from build123d import *

# Parameters (mm, degrees)
SKETCH1_R           = 3.4036
BOSS_EXTRUDE1_DEPTH = 304.8


with BuildPart() as part:
    # Sketch1 → Boss-Extrude1 (new body, symmetric)
    with BuildSketch(Plane.XY):
        with BuildLine():
            Line((-39.878, 16.891), (-39.878, 4.7625))
            ThreePointArc((-39.878, 4.7625), (-39.654815367, 4.223684633), (-39.116, 4.0005))
            Line((-39.116, 4.0005), (-36.1442, 4.0005))
            ThreePointArc((-36.1442, 4.0005), (-35.605384633, 4.223684633), (-35.3822, 4.7625))
            Line((-35.3822, 4.7625), (-35.3822, 10.2235))
            ThreePointArc((-35.3822, 10.2235), (-34.911804775, 10.927496204), (-34.081384633, 10.762315367))
            Line((-34.081384633, 10.762315367), (-28.513059555, 5.19399029))
            ThreePointArc((-28.513059555, 5.19399029), (-27.863348265, 4.221628629), (-27.6352, 3.074649845))
            Line((-27.6352, 3.074649845), (-27.6352, -3.074649845))
            ThreePointArc((-27.6352, -3.074649845), (-27.863348265, -4.221628629), (-28.513059555, -5.19399029))
            Line((-28.513059555, -5.19399029), (-34.081384633, -10.762315367))
            ThreePointArc((-34.081384633, -10.762315367), (-34.911804775, -10.927496204), (-35.3822, -10.2235))
            Line((-35.3822, -10.2235), (-35.3822, -4.7625))
            ThreePointArc((-35.3822, -4.7625), (-35.605384633, -4.223684633), (-36.1442, -4.0005))
            Line((-36.1442, -4.0005), (-39.116, -4.0005))
            ThreePointArc((-39.116, -4.0005), (-39.654815367, -4.223684633), (-39.878, -4.7625))
            Line((-39.878, -4.7625), (-39.878, -16.891))
            ThreePointArc((-39.878, -16.891), (-38.985261469, -19.046261469), (-36.83, -19.939))
            Line((-36.83, -19.939), (-24.7015, -19.939))
            ThreePointArc((-24.7015, -19.939), (-24.162684633, -19.715815367), (-23.9395, -19.177))
            Line((-23.9395, -19.177), (-23.9395, -16.2052))
            ThreePointArc((-23.9395, -16.2052), (-24.162684633, -15.666384633), (-24.7015, -15.4432))
            Line((-24.7015, -15.4432), (-30.1625, -15.4432))
            ThreePointArc((-30.1625, -15.4432), (-30.866496204, -14.972804775), (-30.701315367, -14.142384633))
            Line((-30.701315367, -14.142384633), (-25.13299029, -8.574059555))
            ThreePointArc((-25.13299029, -8.574059555), (-24.160628629, -7.924348265), (-23.013649845, -7.6962))
            Line((-23.013649845, -7.6962), (-16.864350155, -7.6962))
            ThreePointArc((-16.864350155, -7.6962), (-15.717371371, -7.924348265), (-14.74500971, -8.574059555))
            Line((-14.74500971, -8.574059555), (-9.176684633, -14.142384633))
            ThreePointArc((-9.176684633, -14.142384633), (-9.011503796, -14.972804775), (-9.7155, -15.4432))
            Line((-9.7155, -15.4432), (-15.1765, -15.4432))
            ThreePointArc((-15.1765, -15.4432), (-15.715315367, -15.666384633), (-15.9385, -16.2052))
            Line((-15.9385, -16.2052), (-15.9385, -19.177))
            ThreePointArc((-15.9385, -19.177), (-15.715315367, -19.715815367), (-15.1765, -19.939))
            Line((-15.1765, -19.939), (15.1765, -19.939))
            ThreePointArc((15.1765, -19.939), (15.715315367, -19.715815367), (15.9385, -19.177))
            Line((15.9385, -19.177), (15.9385, -16.2052))
            ThreePointArc((15.9385, -16.2052), (15.715315367, -15.666384633), (15.1765, -15.4432))
            Line((15.1765, -15.4432), (9.7155, -15.4432))
            ThreePointArc((9.7155, -15.4432), (9.011503796, -14.972804775), (9.176684633, -14.142384633))
            Line((9.176684633, -14.142384633), (14.74500971, -8.574059555))
            ThreePointArc((14.74500971, -8.574059555), (15.717371371, -7.924348265), (16.864350155, -7.6962))
            Line((16.864350155, -7.6962), (23.013649845, -7.6962))
            ThreePointArc((23.013649845, -7.6962), (24.160628629, -7.924348265), (25.13299029, -8.574059555))
            Line((25.13299029, -8.574059555), (30.701315367, -14.142384633))
            ThreePointArc((30.701315367, -14.142384633), (30.866496204, -14.972804775), (30.1625, -15.4432))
            Line((30.1625, -15.4432), (24.7015, -15.4432))
            ThreePointArc((24.7015, -15.4432), (24.162684633, -15.666384633), (23.9395, -16.2052))
            Line((23.9395, -16.2052), (23.9395, -19.177))
            ThreePointArc((23.9395, -19.177), (24.162684633, -19.715815367), (24.7015, -19.939))
            Line((24.7015, -19.939), (36.83, -19.939))
            ThreePointArc((36.83, -19.939), (38.985261469, -19.046261469), (39.878, -16.891))
            Line((39.878, -16.891), (39.878, -4.7625))
            ThreePointArc((39.878, -4.7625), (39.654815367, -4.223684633), (39.116, -4.0005))
            Line((39.116, -4.0005), (36.1442, -4.0005))
            ThreePointArc((36.1442, -4.0005), (35.605384633, -4.223684633), (35.3822, -4.7625))
            Line((35.3822, -4.7625), (35.3822, -10.2235))
            ThreePointArc((35.3822, -10.2235), (34.911804775, -10.927496204), (34.081384633, -10.762315367))
            Line((34.081384633, -10.762315367), (28.513059555, -5.19399029))
            ThreePointArc((28.513059555, -5.19399029), (27.863348265, -4.221628629), (27.6352, -3.074649845))
            Line((27.6352, -3.074649845), (27.6352, 3.074649845))
            ThreePointArc((27.6352, 3.074649845), (27.863348265, 4.221628629), (28.513059555, 5.19399029))
            Line((28.513059555, 5.19399029), (34.081384633, 10.762315367))
            ThreePointArc((34.081384633, 10.762315367), (34.911804775, 10.927496204), (35.3822, 10.2235))
            Line((35.3822, 10.2235), (35.3822, 4.7625))
            ThreePointArc((35.3822, 4.7625), (35.605384633, 4.223684633), (36.1442, 4.0005))
            Line((36.1442, 4.0005), (39.116, 4.0005))
            ThreePointArc((39.116, 4.0005), (39.654815367, 4.223684633), (39.878, 4.7625))
            Line((39.878, 4.7625), (39.878, 16.891))
            ThreePointArc((39.878, 16.891), (38.985261469, 19.046261469), (36.83, 19.939))
            Line((36.83, 19.939), (24.7015, 19.939))
            ThreePointArc((24.7015, 19.939), (24.162684633, 19.715815367), (23.9395, 19.177))
            Line((23.9395, 19.177), (23.9395, 16.2052))
            ThreePointArc((23.9395, 16.2052), (24.162684633, 15.666384633), (24.7015, 15.4432))
            Line((24.7015, 15.4432), (30.1625, 15.4432))
            ThreePointArc((30.1625, 15.4432), (30.866496204, 14.972804775), (30.701315367, 14.142384633))
            Line((30.701315367, 14.142384633), (25.13299029, 8.574059555))
            ThreePointArc((25.13299029, 8.574059555), (24.160628629, 7.924348265), (23.013649845, 7.6962))
            Line((23.013649845, 7.6962), (16.864350155, 7.6962))
            ThreePointArc((16.864350155, 7.6962), (15.717371371, 7.924348265), (14.74500971, 8.574059555))
            Line((14.74500971, 8.574059555), (9.176684633, 14.142384633))
            ThreePointArc((9.176684633, 14.142384633), (9.011503796, 14.972804775), (9.7155, 15.4432))
            Line((9.7155, 15.4432), (15.1765, 15.4432))
            ThreePointArc((15.1765, 15.4432), (15.715315367, 15.666384633), (15.9385, 16.2052))
            Line((15.9385, 16.2052), (15.9385, 19.177))
            ThreePointArc((15.9385, 19.177), (15.715315367, 19.715815367), (15.1765, 19.939))
            Line((15.1765, 19.939), (-15.1765, 19.939))
            ThreePointArc((-15.1765, 19.939), (-15.715315367, 19.715815367), (-15.9385, 19.177))
            Line((-15.9385, 19.177), (-15.9385, 16.2052))
            ThreePointArc((-15.9385, 16.2052), (-15.715315367, 15.666384633), (-15.1765, 15.4432))
            Line((-15.1765, 15.4432), (-9.7155, 15.4432))
            ThreePointArc((-9.7155, 15.4432), (-9.011503796, 14.972804775), (-9.176684633, 14.142384633))
            Line((-9.176684633, 14.142384633), (-14.74500971, 8.574059555))
            ThreePointArc((-14.74500971, 8.574059555), (-15.717371371, 7.924348265), (-16.864350155, 7.6962))
            Line((-16.864350155, 7.6962), (-23.013649845, 7.6962))
            ThreePointArc((-23.013649845, 7.6962), (-24.160628629, 7.924348265), (-25.13299029, 8.574059555))
            Line((-25.13299029, 8.574059555), (-30.701315367, 14.142384633))
            ThreePointArc((-30.701315367, 14.142384633), (-30.866496204, 14.972804775), (-30.1625, 15.4432))
            Line((-30.1625, 15.4432), (-24.7015, 15.4432))
            ThreePointArc((-24.7015, 15.4432), (-24.162684633, 15.666384633), (-23.9395, 16.2052))
            Line((-23.9395, 16.2052), (-23.9395, 19.177))
            ThreePointArc((-23.9395, 19.177), (-24.162684633, 19.715815367), (-24.7015, 19.939))
            Line((-24.7015, 19.939), (-36.83, 19.939))
            ThreePointArc((-36.83, 19.939), (-38.985261469, 19.046261469), (-39.878, 16.891))
        make_face()
        with Locations((-19.939, 0)):
            Circle(SKETCH1_R, mode=Mode.SUBTRACT)
        with Locations((19.939, 0)):
            Circle(SKETCH1_R, mode=Mode.SUBTRACT)
        with BuildLine():
            Line((-12.2428, 3.074649845), (-12.2428, -3.074649845))
            ThreePointArc((-12.2428, -3.074649845), (-12.014651735, -4.221628629), (-11.364940445, -5.19399029))
            Line((-11.364940445, -5.19399029), (-1.904671503, -14.654259232))
            ThreePointArc((-1.904671503, -14.654259232), (0, -15.4432), (1.904671503, -14.654259232))
            Line((1.904671503, -14.654259232), (11.364940445, -5.19399029))
            ThreePointArc((11.364940445, -5.19399029), (12.014651735, -4.221628629), (12.2428, -3.074649845))
            Line((12.2428, -3.074649845), (12.2428, 3.074649845))
            ThreePointArc((12.2428, 3.074649845), (12.014651735, 4.221628629), (11.364940445, 5.19399029))
            Line((11.364940445, 5.19399029), (1.904671503, 14.654259232))
            ThreePointArc((1.904671503, 14.654259232), (0, 15.4432), (-1.904671503, 14.654259232))
            Line((-1.904671503, 14.654259232), (-11.364940445, 5.19399029))
            ThreePointArc((-11.364940445, 5.19399029), (-12.014651735, 4.221628629), (-12.2428, 3.074649845))
        make_face(mode=Mode.SUBTRACT)
    extrude(amount=BOSS_EXTRUDE1_DEPTH, both=True)


solid = part.part
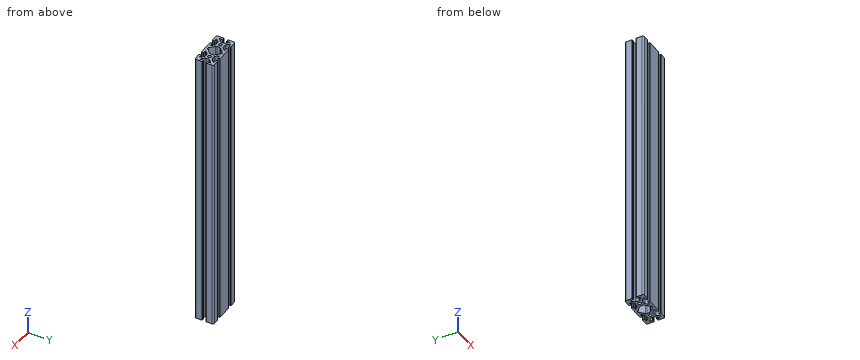
Model file for the job. Use its own axes, mm. Give positions to 0.01 mm unless a question says otherwise; leave off trailing zeros.
Item 1: Drill centre lines: line 1 along X through (y, z) = (-16, -54); line 2 along Y through (x, z) = (32, -231); line 3 along X through (y, z) = (2, 209) (3 decimals). Where is each one in solid material? Low to high.
Check values:
line 1: x = -39.88 to -23.97, -15.91 to 15.91, 23.97 to 39.88
line 2: y = -19.94 to -8.68, 8.68 to 19.94
line 3: x = -27.635 to -22.693, -17.185 to -12.243, 12.243 to 17.185, 22.693 to 27.635
Item 2: Slice it at A-A (z = 227). Give the number of separate pieces and of enclosed holes in the cut face, plus the area to 3 significant figures.
Check values:
separate pieces: 1
enclosed holes: 3
area: 1,620 mm2
Item 3: Drop flat-ended pins along their axis: P1, Ø7, axis at x = -20, z = 100, coming from the -Y side; P2, Ø1.5, axis at y = 18.5, z = -103.5, coming from the +X side; P3, Ø0.9, axis at x = -38.5, z = -22, coming from the -Y side; P4, Ø2.5, axis at y = 18, z = -117, coming from the +X side. Give the stop position or say it passes through.
Check values:
P1: stops at y = -7.74
P2: stops at x = 39.75
P3: stops at y = -19.68
P4: stops at x = 39.88
